from build123d import *

# Parameters (mm, degrees)
SKETCH_2_W               = 52
SKETCH_2_H               = 120
EXTRUDE_1_DEPTH          = 7.5
SKETCH_3_R               = 11.1
EXTRUDE_2_DEPTH          = 60
CUT_EXTRUDE_1_DEPTH      = 81.007562143
CUT_EXTRUDE_1_DEPTH_BACK = 81.007562143
SKETCH_4_W               = 8.2
SKETCH_4_H               = 8.069924866
SKETCH_5_W               = 10.2
SKETCH_5_H               = 26.140993965
CUT_EXTRUDE_2_DEPTH      = 70
SKETCH_6_R               = 4.9
EXTRUDE_3_DEPTH          = 25
EXTRUDE_4_DEPTH          = 120
CUT_EXTRUDE_3_DEPTH      = 104.044523


with BuildPart() as part:
    # 스케치2 → 보스-돌출1 (new, symmetric)
    with BuildSketch(Plane(origin=(0, 0, 0), x_dir=(1, 0, 0), z_dir=(0, 1, 0))):
        Rectangle(SKETCH_2_W, SKETCH_2_H)
    extrude(amount=EXTRUDE_1_DEPTH, both=True)

    # 스케치3 → 보스-돌출2 (add, symmetric)
    with BuildSketch(Plane.XY):
        with BuildLine():
            Line((-26, 32.5), (-26, 7.5))
            Line((-26, 7.5), (26, 7.5))
            Line((26, 7.5), (26, 32.5))
            Line((26, 32.5), (9.6493822, 43.219015699))
            ThreePointArc((9.6493822, 43.219015699), (0, 46.1), (-9.6493822, 43.219015699))
            Line((-9.6493822, 43.219015699), (-26, 32.5))
        make_face()
        with Locations((0, 28.5)):
            Circle(SKETCH_3_R, mode=Mode.SUBTRACT)
    extrude(amount=EXTRUDE_2_DEPTH, both=True)

    # 스케치4 → 컷-돌출1 (cut, two sides: drawn at the far end of the back side and taken through both)
    with BuildSketch(Plane.XY.offset(-CUT_EXTRUDE_1_DEPTH_BACK)):
        with Locations((0, 42.85)):
            Rectangle(SKETCH_4_W, SKETCH_4_H)
    extrude(amount=CUT_EXTRUDE_1_DEPTH + CUT_EXTRUDE_1_DEPTH_BACK, mode=Mode.SUBTRACT)

    # 스케치5 → 컷-돌출2 (cut)
    with BuildSketch(Plane.XY.offset(60)):
        with Locations((0, 5.570496982)):
            Rectangle(SKETCH_5_W, SKETCH_5_H)
    extrude(amount=-CUT_EXTRUDE_2_DEPTH, mode=Mode.SUBTRACT)

    # 스케치6 → 보스-돌출3 (add)
    with BuildSketch(Plane(origin=(0, 0, -60), x_dir=(-1, 0, 0), z_dir=(0, 0, -1))):
        with Locations(Location((13.5, 14.5, 0), (0, 0, 180))):
            Circle(SKETCH_6_R)
        with Locations(Location((-13.5, 14.5, 0), (0, 0, 180))):
            Circle(SKETCH_6_R)
    extrude(amount=EXTRUDE_3_DEPTH)

    # 스케치9 → 보스-돌출4 (add)
    with BuildSketch(Plane.XY.offset(60)):
        Polygon((4.1, 45.615782191), (6.978359415, 44.657428628), (26, 32.5), (26, 45.615782191), align=None)
        Polygon((-26, 45.615782191), (-4.1, 45.615782191), (-6.978359415, 44.657428628), (-26, 32.5), align=None)
    extrude(amount=-EXTRUDE_4_DEPTH)

    # 스케치13 → 컷-돌출3 (cut)
    with BuildSketch(Plane.XY.offset(60)):
        Polygon((26, 38.615782191), (16, 38.615782191), (16, 42.615782191), (12.5, 42.615782191), (12.5, 25.615782191), (16.116710555, 25.615782191), (16.116710555, 29.615782191), (26, 29.615782191), align=None)
    extrude(amount=-CUT_EXTRUDE_3_DEPTH, mode=Mode.SUBTRACT)


solid = part.part
Could you check a few things on this model? Use its own coordinates, in mm. A direction names the side the tool comes from. Give positions to 0.01 mm unless a question says otherwise; leave off trailing zeros. Write each loop counter-clockwise with the first axis right and the second up, starting at its lowest first coordinate (ties: lowest second). Pieces come first, ordered by that corner, then holes. Notation, with made-up numbers: (-30.75, -2) -> (19.25, -2) arc R17 ccw to (19.25, 10) -> close; hole circle Ø9 at (30.5, 55.25). An arc over 180 degrees is marked (long way). Answer as CSV lines item,"result". Start each with the question number.
(1) If we section it at B-B, the plane z = -56.5: Write out the boundary of the cut face in (x, y), and give its area (3 significant figures).
(2) If we section it at C-C, the plane x = 22: Write out the boundary of the cut face in (y, z).
(3) I'm going to push flat-ended pins straight in: pin 1 Ø6 at (x, z) = (4, -30.5) entering from +Y; pin 2 Ø15.5 at (x, y) = (12, 29.5) entering from -Z; pin 3 Ø5 at (x, y) = (-2, 9.5) entering from +Z. Where does each tip first touch, or does it pass through?
(4) If we section it at D-D, the plane z = 13: Write out the boundary of the cut face in (x, y), and give its area (3 significant figures).
(5) Which directions (+Z, -Z, +X, -X, +Y, -Y) give clear straight access to the entire face, cutting with the end or side of a thin tool? Please do faces 1 (the face through (12.5, 34, 9)), 2 (the face through (-4.1, 42, -1)), 3 (the face through (-5.1, 5, 25)), 4 (the face through (21, 38.616, 9)).
(6) If we mould it in two halves opening along Y, with no side actions, what happens to faces 5 (the face through (14, 25.616, 9)), 6 (the face through (18.026, 16.377, -72.325)), 7 (the face through (-14, 14, -85))? For each: +Y half, -Y half, draft (parallel to the pull), parting line (faces both ways), or undercut.
(7) If we section it at A-A, the plane y = 14.5: Write out the boundary of the cut face in (x, z).
(8) Please list where these lines run through material, in increasing order: line 1 (X direction, y = 28.5, z = 14); line 2 (X direction, y = 13.5, z = 11); line 3 (Y direction, x = 20, z = -7).
Answer list:
1,outline,"(-26, -7.5) -> (26, -7.5) -> (26, 45.62) -> (4.1, 45.62) -> (4.1, 38.82) arc R11.1 cw (long way) to (-4.1, 38.82) -> (-4.1, 45.62) -> (-26, 45.62) -> close"
1,area,"2,320 mm^2"
2,outline,"(-7.5, -60) -> (45.62, -60) -> (45.62, 60) -> (38.62, 60) -> (38.62, -44.04) -> (29.62, -44.04) -> (29.62, 60) -> (-7.5, 60) -> close"
3,pin 1,"y = 45.62"
3,pin 2,"z = -60"
3,pin 3,"z = -10"
4,outline,"(-26, -7.5) -> (-5.1, -7.5) -> (-5.1, 18.64) arc R11.1 cw to (-4.1, 38.82) -> (-4.1, 45.62) -> (-26, 45.62) -> close; (4.1, 38.82) arc R11.1 cw to (5.1, 18.64) -> (5.1, -7.5) -> (26, -7.5) -> (26, 29.62) -> (16.12, 29.62) -> (16.12, 25.62) -> (12.5, 25.62) -> (12.5, 42.62) -> (16, 42.62) -> (16, 38.62) -> (26, 38.62) -> (26, 45.62) -> (4.1, 45.62) -> close"
4,area,"1,920 mm^2"
5,face 1,"+Z"
5,face 2,"+Z, -Z, +Y"
5,face 3,"+Z, -Y"
5,face 4,"+Z, +X"
6,face 5,"undercut"
6,face 6,"parting line"
6,face 7,"draft"
7,outline,"(-26, -60) -> (-18.4, -60) -> (-18.4, -85) -> (-8.6, -85) -> (-8.6, -60) -> (8.6, -60) -> (8.6, -85) -> (18.4, -85) -> (18.4, -60) -> (26, -60) -> (26, 60) -> (5.1, 60) -> (5.1, -10) -> (-5.1, -10) -> (-5.1, 60) -> (-26, 60) -> close"
8,line 1,"-26 to -11.1, 11.1 to 12.5, 16.12 to 26"
8,line 2,"-26 to -5.1, 5.1 to 26"
8,line 3,"-7.5 to 29.62, 38.62 to 45.62"
